Check sheet for the modelled part. Datum: model origin and axes. Units: mm. Face numbers are marked on the shaded views. A direction names the side the tool comes from. Give positions to 0.01 mm unless a question says otherwise; leave off trailing zeros. Order: outer loops, then holes, each group sorted by start corner. A loop starts at its lowest first (then second) coordinate and runs counter-clockwise, first axis right, second up. Notation, with made-up numbers: (78, 60.25) -> (108, 60.25) arc R9 cw to (108, 74.25) -> close; hole circle Ø7 at (-15.75, 87.5). An arc over 180 degrees is marked (long way). One line per question, with ' | ' between items. Start each with the question number.
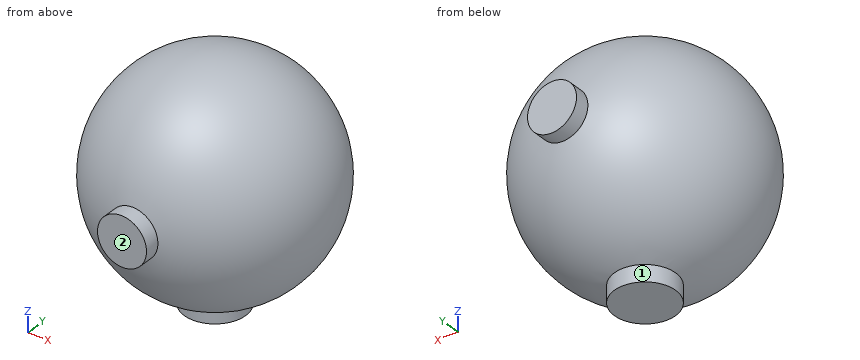
Autodesk Inventor part; units mm, degrees
ref_plane "YZ Plane" through (0, 0, 0) normal (1, 0, 0) x (0, 1, 0)
sketch "スケッチ1" plane through (0, 0, 0) normal (0, 0, 1) x (1, 0, 0)
  arc A0 (0, 90) -> (0, -90) centre (0, 0) ccw
  line L0 (0, 90) -> (0, -90)
  dimension "d0" = 180
revolve "回転1" add sketch "スケッチ1" angle 360 about axis through (0, 90, 0) along (0, -1, 0)
sketch "スケッチ2" plane through (0, 0, 0) normal (0, 1, 0) x (-1, 0, 0)
  circle A0 centre (0, 0) radius 20
  dimension "d2" = 40
extrude "押し出し1" add sketch "スケッチ2" along normal mid plane 200
sketch "スケッチ3" plane through (0, 0, 0) normal (0, 0, 1) x (1, 0, 0)
  circle A0 centre (0, 0) radius 25
  dimension "d5" = 50
extrude "押し出し2" add sketch "スケッチ3" against normal blind 100
properties part number "HeadY"
1. Cross-section at C-C on y = 0. Record the boundary of the cut face in (x, z), and give its area (3 significant figures).
2. Go/stop test with flat-tipped pins: pin 1 (8 mm diameter, centred on x = -45, z = 66, fed in from +Y); pin 2 (1.5 mm diameter, centred on y = 55, z = -24.5, fed in from -X); pin 3 (12 mm diameter, centred on x = -30, y = -33, fed in from -Z). Record where each tip stops, or that it passes through.
3. Cross-section at D-D on y = 62. Record the boundary of the cut face in (x, z), and give its area (3 significant figures).
4. Cross-section at B-B on x = 0. Record the boundary of the cut face in (y, z).
5. Scan lines: probe 1 along Y at (x, z) = (-20.5, -73); probe 2 along Y at (x, z) = (72, 24); probe 3 along X at (y, z) = (46.5, 38.5). Record each from-to range of solid material in increasing order.
6. Tool access check on the marked faces 1 and 2. Record the directions out of +Z, -Z, +X, -X, +Y, -Y that give a thin tool (end or side, any length) a straight path to the whole face; none if there is none.
7. Cross-section at A-A on z = 0. Record the boundary of the cut face in (x, y), and give its area (3 significant figures).
Response values:
1) outline: (-25, -100) -> (25, -100) -> (25, -86.46) arc R90 ccw (long way) to (-25, -86.46) -> close | area: 26,000 mm²
2) pin 1: stops at y = 48.39 | pin 2: stops at x = -67.56 | pin 3: stops at z = -81.3
3) outline: circle Ø130.48 at (0, 0) | area: 13,400 mm²
4) outline: (-100, -20) -> (-87.75, -20) arc R90 ccw to (-25, -86.46) -> (-25, -100) -> (25, -100) -> (25, -86.46) arc R90 ccw to (87.75, -20) -> (100, -20) -> (100, 20) -> (87.75, 20) arc R90 ccw to (-87.75, 20) -> (-100, 20) -> close
5) probe 1: y = -48.48 to 48.48 | probe 2: y = -48.37 to 48.37 | probe 3: x = -66.75 to 66.75
6) face 1: -Z | face 2: +Z, -Z, +X, -X, -Y
7) outline: (-20, -100) -> (20, -100) -> (20, -87.75) arc R90 ccw to (20, 87.75) -> (20, 100) -> (-20, 100) -> (-20, 87.75) arc R90 ccw to (-20, -87.75) -> close | area: 26,300 mm²
